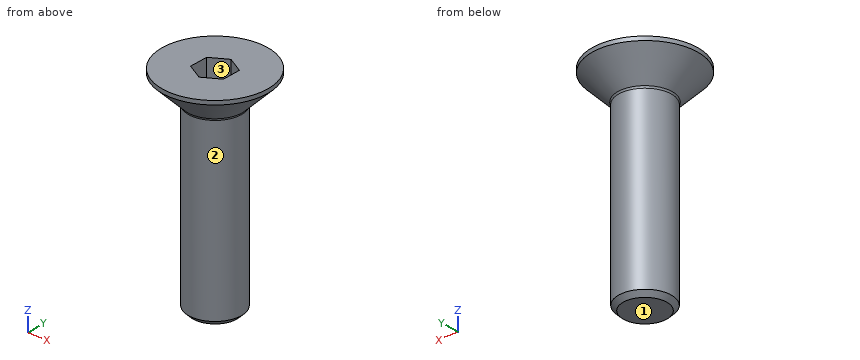
Autodesk Inventor part; units mm, degrees
ref_plane "MSC_PF1" through (0, 0, 0) normal (1, 0, 0) x (0, 1, 0)
ref_plane "MSC_PT1" through (0, 0, 0) normal (0, 0, -1) x (-1, 0, 0)
ref_plane "YZ Plane" through (0, 0, 0) normal (1, 0, 0) x (0, 1, 0)
sketch "Sketch1" plane through (0, 0, 0) normal (0, 1, 0) x (-1, 0, 0)
  point P0 (0, 0)
sketch "Sketch2" plane through (0, 0, 0) normal (0, 1, 0) x (-1, 0, 0)
  line L0 (-2, -16) -> (0, -16)
  line L1 (-2, -2.3) -> (-2, -16)
  line L2 (-4, -0.3) -> (-2, -2.3)
  line L3 (-4, 0) -> (-4, -0.3)
  line L4 (0, 0) -> (-4, 0)
  line L5 (0, -16) -> (0, 0)
  line L6 (0, -16) -> (0, 0)
  line L7 (0, -19.2) -> (0, 3.2)
  line L8 (0.8, 0) -> (-4.8, 0)
  dimension "d3" = 4
  dimension "d5" = 2
  dimension "d7" = 16
  dimension "ParC" = 0.3
  dimension "d22" = 0
  dimension "d23" = 0
  dimension "d43" = 45
revolve "Revolution1" add sketch "Sketch2" angle 360 about axis through (0, 0, -16) along (0, 0, -1)
sketch "Sketch3" plane through (0, 0, 0) normal (0, 0, 1) x (1, 0, 0)
  line L0 (-1.25, 0.7217) -> (-1.25, -0.7217)
  line L1 (0, 1.4434) -> (-1.25, 0.7217)
  line L2 (1.25, 0.7217) -> (0, 1.4434)
  line L3 (1.25, -0.7217) -> (1.25, 0.7217)
  line L4 (0, -1.4434) -> (1.25, -0.7217)
  line L5 (-1.25, -0.7217) -> (0, -1.4434)
  circle A0 centre (0, 0) radius 1.25 construction
  circle A1 centre (0, 0) radius 2 construction
  dimension "d11" = 2.5
  dimension "d13" = 120
  dimension "d15" = 120
extrude "Extrusion1" cut sketch "Sketch3" against normal blind 1.8
fillet "Fillet1" radius 0.2 1 edges at (-2, 0, -2.3)
chamfer "Chamfer1" distance 0.35 angle 45 1 edges at (-2, 0, -16) measured on face at (-0.9288, -1.7713, -11.4609)
thread "Thread1"
ref_plane "MSC_PF1" through (0, 0, 0) normal (1, 0, 0) x (0, 1, 0)
ref_plane "MSC_PT1" through (0, 0, 0) normal (0, 0, -1) x (-1, 0, 0)
equation "\"d3\" = 0.5 * dk"
equation "\"d5\" = 0.5 * NND"
equation "\"d7\" = NLG"
equation "\"d43\" = 0.5 * ang"
equation "\"d18\" = r"
equation "\"d19\" = 0.5 * PTC"
equation "\"d39\" = 0.5 * PTC"
equation "\"d11\" = ParS"
equation "\"d16\" = ParT"
equation "\"NND\" = 4"
equation "\"PTC\" = 0.7"
equation "\"dk\" = 8"
equation "\"ParK\" = 2.3"
equation "\"ParS\" = 2.5"
equation "\"ParT\" = 1.8"
equation "\"r\" = 0.2"
equation "\"NLG\" = 16"
equation "\"ang\" = 90deg"
equation "\"THREADDIA\" = NND"
properties part number "DIN 7991 - M4x16" material "Steel, Mild"
The listing builds one solid part. Answer for the finished solid, in the listing's coordinates (mm). Face numbers are marked on the shaded views. Coordinates: 2 decimals unless noted, no trailing zeros. Loops run counter-clockwise (first coordinate to the right, second up) from the corner with the lowest first, then second, coordinate; pieces in that order, holes last. Notation, with made-up numbers: (-21.75, 31) -> (32.25, 31) arc R25 ccw to (32.25, 46) -> close; hole circle Ø3 at (21.25, -16). An arc over 180 degrees is marked (long way). Return JSON: item names as keys, results as strings. Group by question number.
(1) A cutting plane is placed at A-A on z = -8.75. Write down the section's boundary in (x, y), and give its area (3 significant figures).
(2) Given pin 1 Ø1.5 at (x, y) = (-3, 0.5) entering from -Z; pin 2 Ø4 at (y, z) = (1, -12.5) entering from -X; pin 3 Ø0.7 at (y, z) = (0.5, -1.5) entering from +X, each flat-ended and moving along its own axis, determine where each tip first touches the part or whether it passes through.
(3) Determine the mould class of the marked faces 1, 2 and 3 for opening direction Y: released by +Y, released by -Y, zero draft, split by the parting line, or undercut.
(4) Find the intervals of material crossed by probe 1 along Z at (x, y) = (0.25, -0.75); probe 2 along Y at (x, z) = (0, -2.75); probe 3 along Z at (x, y) = (-1.5, -1.5), in increasing order. Write a range as from..to.
The answers:
{
 "1": {"outline": "circle Ø4 at (0, 0)", "area": "12.6 mm^2"},
 "2": {"pin 1": "stops at z = -2.01", "pin 2": "stops at x = -2", "pin 3": "stops at x = 3.11"},
 "3": {"face 1": "zero draft", "face 2": "split by the parting line", "face 3": "undercut"},
 "4": {"probe 1": "z = -16..-1.8", "probe 2": "y = -2..2", "probe 3": "z = -2.18..0"}
}
